Geometry check sheet. Reference: the model listing, model coordinates, mm. Face numbers are marked on the shaded views. A direction names the side the tool comes from. Round coordinates to 2 decimals unless told otherwise and drop trailing zeros. Order: outer loops, then holes, each group sorted by start corner. A loop starts at its lowest first (then second) coordinate and runs counter-clockwise, first axis right, second up.
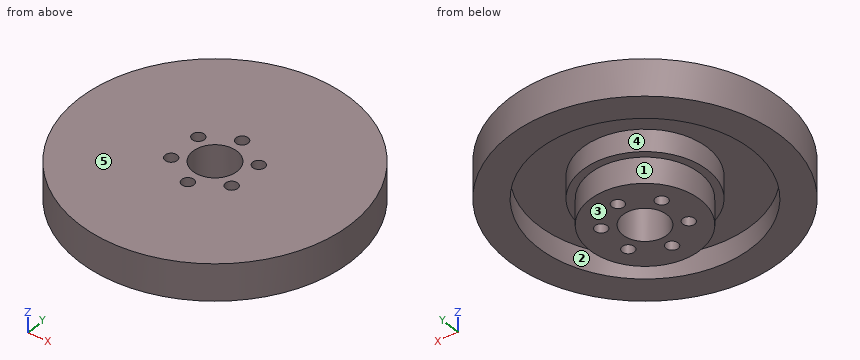
Autodesk Inventor part; units mm, degrees
ref_plane "YZ Plane" through (0, 0, 0) normal (1, 0, 0) x (0, 1, 0)
ref_plane "XZ Plane" through (0, 0, 0) normal (0, 1, 0) x (-1, 0, 0)
ref_plane "XY Plane" through (0, 0, 0) normal (0, 0, 1) x (1, 0, 0)
sketch "Sketch1" plane through (0, 0, 0) normal (0, 0, 1) x (1, 0, 0)
  circle A0 centre (0, 0) radius 37
  dimension "d0" = 74
extrude "Extrusion1" add sketch "Sketch1" along normal blind 10
sketch "Sketch4" plane through (0, 0, 0) normal (0, 0, -1) x (-1, 0, 0)
  circle A0 centre (0, 0) radius 29
  circle A1 centre (0, 0) radius 17
  circle A2 centre (0, 0) radius 37
  dimension "d5" = 8
  dimension "d6" = 34
extrude "Extrusion3" cut sketch "Sketch4" against normal blind 6 contours A0
sketch "Sketch6" plane through (0, 0, 0) normal (0, 0, -1) x (-1, 0, 0)
  circle A0 centre (0, 0) radius 15
  dimension "d9" = 30
extrude "Extrusion4" add sketch "Sketch6" along normal blind 7
sketch "Sketch8" plane through (0, 0, -7) normal (0, 0, -1) x (-1, 0, 0)
  circle A0 centre (0, 0) radius 9.5
  circle A1 centre (0, 9.5) radius 1.65
  circle A2 centre (-8.2272, 4.75) radius 1.65
  circle A3 centre (-8.2272, -4.75) radius 1.65
  circle A4 centre (0, 0) radius 6
  circle A5 centre (0, -9.5) radius 1.65
  circle A6 centre (8.2272, -4.75) radius 1.65
  circle A7 centre (8.2272, 4.75) radius 1.65
  dimension "d16" = 19
  dimension "d17" = 3.3
  dimension "d20" = 360
  dimension "d24" = 12
extrude "Extrusion6" cut sketch "Sketch8" against normal through all contours A7 A0 | A0 A7 | A6 A0 | A0 A6 | A1 A0 | A0 A1 | A5 A0 | A0 A5 | A2 A0 | A0 A2 | A3 A0 | A0 A3 | A4
properties part number "rotor_hub" material "Aluminum 6061"
(1) Sectioned sample at B-B, the plane y = 0. Record the cut outline in (x, z).
Returned:
outline: (-37, 0) - (-29, 0) - (-29, 6) - (-17, 6) - (-17, 0) - (-15, 0) - (-15, -7) - (-6, -7) - (-6, 10) - (-37, 10) - close; (6, -7) - (15, -7) - (15, 0) - (17, 0) - (17, 6) - (29, 6) - (29, 0) - (37, 0) - (37, 10) - (6, 10) - close
(2) Set-up check for the marked faces 4 and 5: record each of +Z, -Z, +X, -X, +Y, -Y from which the full face is reachable in a straight line by a thin tool's end or side.
Returned:
face 4: -Z
face 5: +Z, +X, -X, +Y, -Y
(3) Depth check by flat-ended pin: P1, Ø2.5, axis at x = -8.23, y = 4.75, coming from the +Z side; P2, Ø10, axis at y = 28.5, z = 3.5, coming from the -X side; P3, Ø2, axis at x = -15, z = 3, coming from the +Y side; P4, Ø6, axis at y = -11.5, z = 4.5, coming from the +X side. Enter the tip coordinate at first touch or a pass-through.
Returned:
P1: passes through
P2: stops at x = -28.58
P3: stops at y = 34.25
P4: stops at x = 36.01
(4) Sectioned sample at A-A, the plane z = -2.5. Record the cut outline in (x, y), and give its area (3 significant figures).
Returned:
outline: circle Ø30 at (0, 0); hole circle Ø3.3 at (-8.23, -4.75); hole circle Ø3.3 at (-8.23, 4.75); hole circle Ø12 at (0, 0); hole circle Ø3.3 at (0, -9.5); hole circle Ø3.3 at (0, 9.5); hole circle Ø3.3 at (8.23, -4.75); hole circle Ø3.3 at (8.23, 4.75)
area: 542 mm2
(5) Draft check along Y on the marked faces 1, 2 and 3. Enter one of: released by +Y, released by -Y, zero draft, split by the parting line, or undercut.
Returned:
face 1: split by the parting line
face 2: undercut
face 3: zero draft
(6) Material ranges on line 1 (Y direction, x = 0, z = 3.75); line 2 (X direction, y = 4.75, z = 0.5); line 3 (Y direction, x = 10, z = 5.75), recorded low to high.
Returned:
line 1: y = -37 to -29, -17 to -11.15, -7.85 to -6, 6 to 7.85, 11.15 to 17, 29 to 37
line 2: x = -36.69 to -28.61, -16.32 to -9.88, -6.58 to -3.67, 3.67 to 6.58, 9.88 to 16.32, 28.61 to 36.69
line 3: y = -35.62 to -27.22, -13.75 to 13.75, 27.22 to 35.62
(7) Sectioned sample at C-C, the plane x = 9. Record the cut outline in (y, z).
Returned:
outline: (-35.89, 0) - (-27.57, 0) - (-27.57, 6) - (-14.42, 6) - (-14.42, 0) - (-12, 0) - (-12, -7) - (-6.21, -7) - (-6.21, 10) - (-35.89, 10) - close; (-3.29, -7) - (3.29, -7) - (3.29, 10) - (-3.29, 10) - close; (6.21, -7) - (12, -7) - (12, 0) - (14.42, 0) - (14.42, 6) - (27.57, 6) - (27.57, 0) - (35.89, 0) - (35.89, 10) - (6.21, 10) - close
(8) Sectioned sample at D-D, the plane y = -9.5. Record the cut outline in (x, z).
Returned:
outline: (-35.76, 0) - (-27.4, 0) - (-27.4, 6) - (-14.1, 6) - (-14.1, 0) - (-11.61, 0) - (-11.61, -7) - (-1.65, -7) - (-1.65, 10) - (-35.76, 10) - close; (1.65, -7) - (11.61, -7) - (11.61, 0) - (14.1, 0) - (14.1, 6) - (27.4, 6) - (27.4, 0) - (35.76, 0) - (35.76, 10) - (1.65, 10) - close
